Source: three-view drawing plus pictorial views. Frame: mm from the lowest corner of the part. A direction names the side the tool comes from. Coordinates: 2 decimals unless noted, no trailing zeros. Order: outer loops, then holes, each group sorted by start corner. A loop starts at its lowest first (then second) coordinate and runs counter-clockwise, first axis right, second up. Notation, with made-up numbers: (-33.75, -7.75) -> (-2.75, -7.75) arc R12 ccw to (-2.75, 4.25) -> close; hole circle Ø1 at (-28.5, 76.25). An arc over 180 degrees is marked (long way). Use one line per item in the form item = value. Start each with the question number.
1) Section query A-A on y = 6. Output: boundary loops of the cut face in (x, z) (1 decimal).
2) Ray query, line 1 along X through (y, z) = (1.5, 2); line 2 along Z through (x, y) = (10, 0.5); line 3 along Z through (x, y) = (1.5, 2.25). Return the intervals inside material, ascending.
3) Section query B-B on x = 11.75. Output: boundary loops of the cut face in (y, z), then the cut area to 3 significant figures.
4) Access query for the marked faces 1, 2, 3 and 4. Directions: +Z, -Z, +X, -X, +Y, -Y. A direction counts if a zero-diameter tool reaches every point of the face in a straight line with its end or side. Return the directions, or none.
5) Section query C-C on z = 6. Output: boundary loops of the cut face in (x, y) (1 decimal).
6) Pin query (flat end, axial travel): pin 1 (2.5 mm diameter, centred on y = 5.5, z = 8.5, fed in from +X) (1 decimal); pin 2 (2 mm diameter, centred on x = 12.5, y = 5.5, fed in from -Z); pin 3 (1.3 mm diameter, centred on x = 2.5, y = 5.5, fed in from +Z). Return the tip coordinate at first contact, or that it passes through.
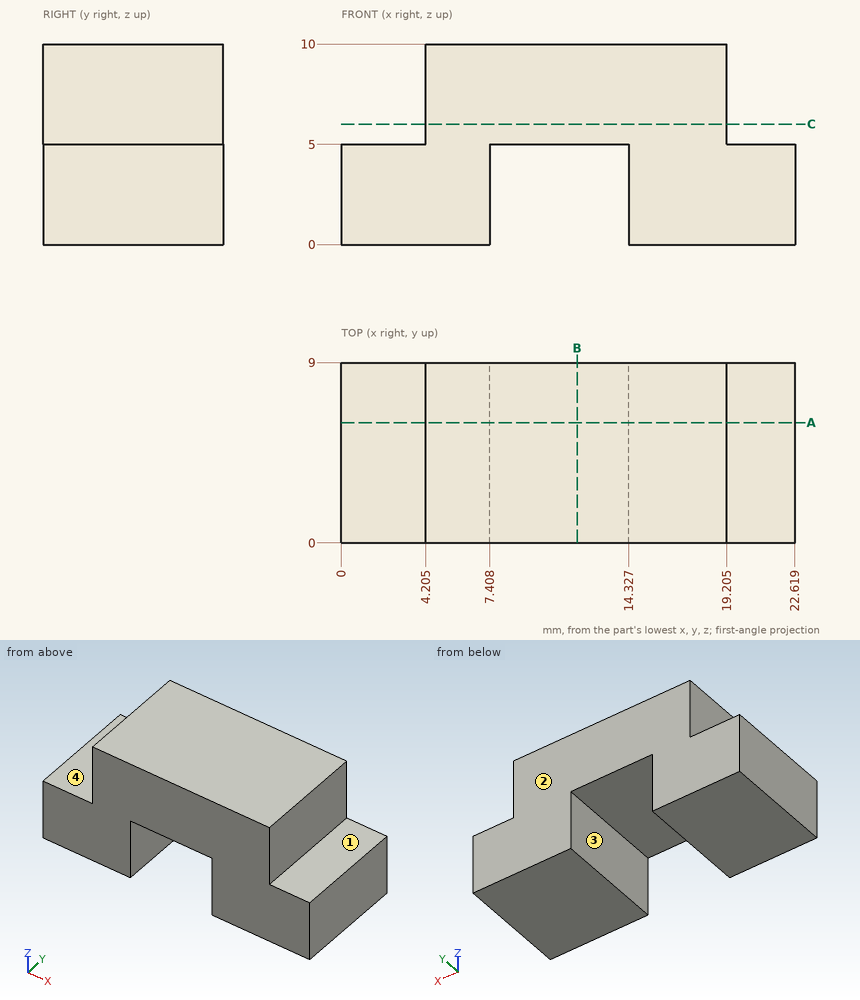
Answers below:
q1.outline = (0, 0) -> (7.4, 0) -> (7.4, 5) -> (14.3, 5) -> (14.3, 0) -> (22.6, 0) -> (22.6, 5) -> (19.2, 5) -> (19.2, 10) -> (4.2, 10) -> (4.2, 5) -> (0, 5) -> close
q2.line_1 = 0 to 7.41, 14.33 to 22.62
q2.line_2 = 5 to 10
q2.line_3 = 0 to 5
q3.outline = (0, 5) -> (9, 5) -> (9, 10) -> (0, 10) -> close
q3.area = 45.0 mm^2
q4.face_1 = +Z, +X, +Y, -Y
q4.face_2 = +Z, -Z, +X, -X, +Y
q4.face_3 = -Z, +Y, -Y
q4.face_4 = +Z, -X, +Y, -Y
q5.outline = (4.2, 0) -> (19.2, 0) -> (19.2, 9) -> (4.2, 9) -> close
q6.pin_1 = 19.2
q6.pin_2 = 5
q6.pin_3 = 5
